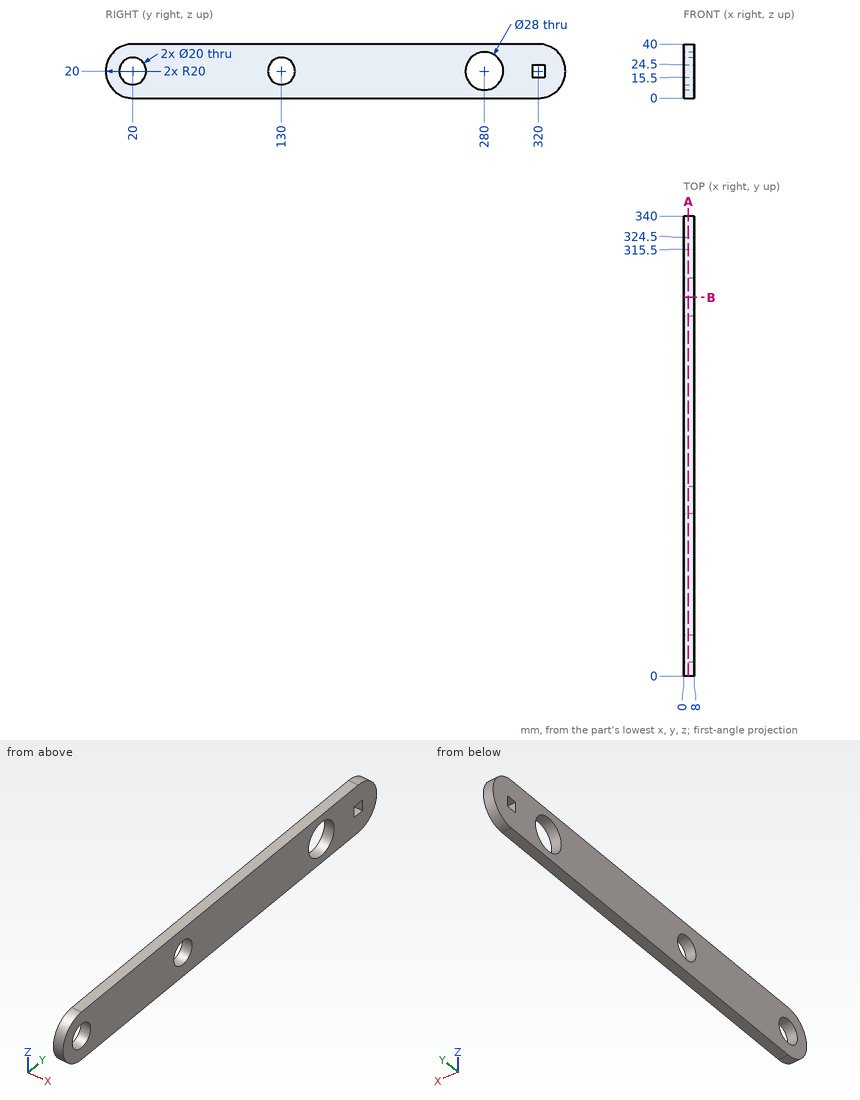
Design review of the part shown in the three views and the two pictorial views. Dimensions are in mm from the part's minimum x, y and z. Round coordinates to 2 decimals unless told otherwise and drop trailing zeros. Loops run counter-clockwise (first coordinate to the right, second up) from the corner with the lowest first, then second, coordinate; pieces in that order, holes last. Notation, with made-up numbers: (-11, 74.5) -> (18, 74.5) arc R25 ccw to (18, 91.5) -> close; hole circle Ø9 at (23.5, 8). An arc over 180 degrees is marked (long way). Answer as CSV lines item,"result".
1) Add section B-B on y = 280. Write out the cut boundary in (x, z), plus the area to 3 significant figures.
Geometry results:
outline,"(0, 0) -> (8, 0) -> (8, 6) -> (0, 6) -> close; (0, 34) -> (8, 34) -> (8, 40) -> (0, 40) -> close"
area,"96.0 mm²"
2) Add section A-A on x = 3.5. Write out the cut boundary in (y, z), plus the area to 3 significant figures.
Geometry results:
outline,"(20, 0) -> (320, 0) arc R20 ccw to (320, 40) -> (20, 40) arc R20 ccw to start; hole circle Ø20 at (20, 20); hole circle Ø20 at (130, 20); hole circle Ø28 at (280, 20); hole (315.5, 15.5) -> (324.5, 15.5) -> (324.5, 24.5) -> (315.5, 24.5) -> close"
area,"11,900 mm²"
3) To check wall thickness, follow line 1 along Y through (x, z) = (3.25, 20); line 2 along Y through (x, z) = (2.25, 22.5); line 3 along Y through (x, z) = (7, 13.5). State the ranges of each line that lie inside material, in increasing order. Write a range as from..to.
Geometry results:
line 1,"y = 0..10, 30..120, 140..266, 294..315.5, 324.5..340"
line 2,"y = 0.16..10.32, 29.68..120.32, 139.68..266.23, 293.77..315.5, 324.5..339.84"
line 3,"y = 1.09..12.4, 27.6..122.4, 137.6..267.6, 292.4..338.91"
4) For P1, Ø1, axis at x = 3, z = 19.5, coming from the -Y side; P2, Ø2, axis at x = 6, z = 20, coming from the +Y side; P3, Ø1, axis at x = 2, z = 29.5, coming from the +Y side, all flat-tipped, find the tip position at first contact; note any pin that passes through.
Geometry results:
P1,"stops at y = 0"
P2,"stops at y = 340"
P3,"stops at y = 337.86"
